Geometry check sheet. Reference: the model listing, model coordinates, mm. A direction names the side the tool comes from. Round coordinates to 2 decimals unless told otherwise and drop trailing zeros. Order: outer loops, then holes, each group sorted by start corner. A loop starts at its lowest first (then second) coordinate and runs counter-clockwise, first axis right, second up. Notation, with made-up numbers: (-4, -39.5) - (25, -39.5) arc R22 cw to (25, -28.5) - close; hole circle Ø8 at (39.25, 58.5). An arc over 180 degrees is marked (long way). One line per question, with ' | ' between items. Start each with the question number.
Q1. Tool access check on faces 5 (the face through (58.859, 3.797, 0.154)), 6 (the face through (19.17, 8, 0.15)), 7 (the face through (21.94, 9.16, 0.15)), 8 (the face through (41.827, 2.465, 0.705)). Record the directions out of +Z, -Z, +X, -X, +Y, -Y that give a thin tool (end or side, any length) a straight path to the whole face; none if there is none.
Q2. Sectioned sample at B-B, the plane x = 45. Enter the section's corners in (y, z).
Q3. Sectioned sample at D-D, the plane x = 53.5. Enter the section's corners in (y, z), then the cut area to 3 significant figures.
Q4. Mould release check, pull along Y, two halves, no side actions. Record for faces 1 (the face through (21, 21, 0)), 2 (the face through (31.86, 24.79, 0.15)), 3 (the face through (15, 3, 0)), 4 (the face through (30, 0, 0)): +Y half, -Y half, draft (parallel to the pull), parting line (faces both ways), or undercut.
Q5. Sectioned sample at A-A, the plane z = 1.5. Enter the section's corners in (x, y).
Q6. Sectioned sample at C-C, the plane z = -8. Enter the section's corners in (x, y).
Q7. Gauge pin test, flat ends, axial feed: P1, Ø3, axis at y = 12, z = -6, coming from the -X side; P2, Ø1, axis at y = 19, z = 7.5, coming from the +X side; P3, Ø5, axis at y = 35.5, z = 4, coming from the -X side; P4, Ø1, axis at x = 46.5, z = 1, coming from the -Y side. Record the tip position at first contact, or that the pin passes through.
Q8. Material ranges on line 1 along Y through (x, z) = (5, 7); line 2 along X through (y, z) = (1.6, 0); line 3 along Y through (x, z) = (43.5, 3.75), recorded low to high.
```python
from build123d import *

# Parameters (mm, degrees)
EXTRUDE_1_DEPTH     = 11
SKETCH_2_R          = 3.25
CUT_EXTRUDE_1_DEPTH = 5
SKETCH_3_R          = 3.25
CUT_EXTRUDE_2_DEPTH = 5
FILLET_1_R          = 4
FILLET_2_R          = 1


with BuildPart() as part:
    # Эскиз1 → Бобышка-Вытянуть1 (new body, symmetric)
    with BuildSketch(Plane.XY):
        Polygon((0, 0), (42.426406871, 42.426406871), (45.961940777, 38.890872965), (20.266663343, 13.195595531), (23.661390163, 5), (60, 5), (60, 0), align=None)
        Polygon((17.142135624, 12.899494937), (21.242640687, 3), (7.242640687, 3), align=None, mode=Mode.SUBTRACT)
    extrude(amount=EXTRUDE_1_DEPTH, both=True)

    # Эскиз2 → Вырез-Вытянуть1 (cut)
    with BuildSketch(Plane(origin=(0, 0, 0), x_dir=(0, 0, 1), z_dir=(-0.707106781, 0.707106781, 0))):
        with Locations(Location((0, 45, 0), (0, 0, 270))):  # turned: the seam where the file's is
            Circle(SKETCH_2_R)
    extrude(amount=-CUT_EXTRUDE_1_DEPTH, mode=Mode.SUBTRACT)

    # Эскиз3 → Вырез-Вытянуть2 (cut)
    with BuildSketch(Plane.XZ):
        with Locations(Location((45, 0, 0), (0, 0, 270))):  # turned: the seam where the file's is
            Circle(SKETCH_3_R)
    extrude(amount=-CUT_EXTRUDE_2_DEPTH, mode=Mode.SUBTRACT)

    # Скругление1
    fillet_1_edges = [part.edges().sort_by_distance(p)[0] for p in [
        (45.961940777, 38.890872965, 0),
        (60, 5, 0),
    ]]
    fillet(fillet_1_edges, radius=FILLET_1_R)

    # Скругление2
    fillet_2_edges = [part.edges().sort_by_distance(p)[0] for p in [
        (17.142135624, 12.899494937, 0),
        (7.242640687, 3, 0),
        (21.242640687, 3, 0),
    ]]
    fillet(fillet_2_edges, radius=FILLET_2_R)


solid = part.part
```
Determined:
1) face 5: +Z, -Z, +X, +Y | face 6: +Z, -Z | face 7: +Z, -Z, +X | face 8: -Y
2) outline: (0, -11) - (5, -11) - (5, -3.25) - (0, -3.25) - close; (0, 3.25) - (5, 3.25) - (5, 11) - (0, 11) - close
3) outline: (0, -11) - (5, -11) - (5, 11) - (0, 11) - close | area: 110 mm2
4) face 1: +Y half | face 2: undercut | face 3: undercut | face 4: -Y half
5) outline: (0, 0) - (42.12, 0) - (42.12, 5) - (23.66, 5) - (20.27, 13.2) - (33.32, 26.25) - (29.78, 29.78) - close; (33.86, 33.86) - (37.39, 30.32) - (43.13, 36.06) arc R4 ccw to (43.13, 41.72) - (42.43, 42.43) - close; (47.88, 0) - (60, 0) - (60, 1) arc R4 ccw to (56, 5) - (47.88, 5) - close; hole (8.95, 4.71) arc R1 ccw to (9.66, 3) - (19.75, 3) arc R1 ccw to (20.67, 4.38) - (17.71, 11.52) arc R1 ccw to (16.08, 11.84) - close
6) outline: (0, 0) - (60, 0) - (60, 1) arc R4 ccw to (56, 5) - (23.66, 5) - (20.27, 13.2) - (43.13, 36.06) arc R4 ccw to (43.13, 41.72) - (42.43, 42.43) - close; hole (8.95, 4.71) arc R1 ccw to (9.66, 3) - (19.75, 3) arc R1 ccw to (20.67, 4.38) - (17.71, 11.52) arc R1 ccw to (16.08, 11.84) - close
7) P1: stops at x = 10.5 | P2: stops at x = 26.57 | P3: stops at x = 33 | P4: passes through
8) line 1: y = 0 to 5 | line 2: x = 1.6 to 41.75, 48.25 to 59.95 | line 3: y = 0 to 5, 36.48 to 41.3
